from build123d import *

# Parameters (mm, degrees)
SLOT_DEPTH      = 26.980762114
SLOT_DEPTH_BACK = 26.980762114
SLOTSKE_W       = 3.5
SLOTSKE_H       = 1.8


with BuildPart() as part:
    # BodySke → Base-Revolve (revolve)
    with BuildSketch(Plane.XY, mode=Mode.PRIVATE) as base_revolve_sk:
        Polygon((0, 0), (0, 4), (1, 5), (24.172, 5), (25, 4.172), (25, 0), align=None)
    revolve(base_revolve_sk.sketch.rotate(Axis((-3.67611336, 0, 0), (1, 0, 0)), 90), axis=Axis((-3.67611336, 0, 0), (1, 0, 0)))

    # SlotSke → Slot (cut, two sides: drawn at the far end of the back side and taken through both)
    with BuildSketch(Plane.XY.offset(-SLOT_DEPTH_BACK)):
        with Locations((1.75, 0)):
            Rectangle(SLOTSKE_W, SLOTSKE_H)
    extrude(amount=SLOT_DEPTH + SLOT_DEPTH_BACK, mode=Mode.SUBTRACT)


solid = part.part
Could you check a few things on this model? Use its own coordinates, in mm. A direction names the side the tool comes from. Give positions to 0.01 mm unless a question says otherwise; leave off trailing zeros. Order: outer loops, then holes, each group sorted by start corner. A loop starts at its lowest first (then second) coordinate and runs counter-clockwise, first axis right, second up.
1. For faces 4 (the flat face through (25, 0, 0)), 5 (the flat face through (3.5, 0, 0)), which set-ups out of +Z, -Z, +X, -X, +Y, -Y let a thin tool reach every point of the face, with its end or its side?
2. Suppose I cut it at C-C (x = 20.25). List the corners of the cut face in (y, z) for me.
3. Will this pin go through, and if not, where does the flat tip stop? P1, Ø1.8, axis at x = 1, z = -0.5, coming from the -Y side.
4. Suppose I cut it at B-B (y = 0). List the corners of the cut face in (x, z) for me, plus the area to 3 significant figures.
5. Suppose I cut it at A-A (z = 0). List the corners of the cut face in (x, y) for me.
6. I need wall thicknesses on L1, parallel to X at y = 0, z = -1; L2, parallel to Y at x = 9.75, z = -3; L3, parallel to Y at x = 6.75, z = -0.25. Which ranges of each line are inside material? Lowest first, please.
7. We'd pull the mould along Y, two halves only. Please class faces 1 (the conical face through (0.2, 4.2, -0.1)), 2 (the flat face through (0, -2, 0)), 3 (the flat face through (2, 0.9, 0)): pulls with the +Y half, pulls with the -Y half, needs draft (parallel to the pull), parting line crosses it, or undercut.
Solved:
1. face 4: +Z, -Z, +X, +Y, -Y
1. face 5: +Z, -Z, -X
2. outline: circle Ø10 at (0, 0)
3. P1: stops at y = -5
4. outline: (3.5, -5) - (24.17, -5) - (25, -4.17) - (25, 4.17) - (24.17, 5) - (3.5, 5) - close
4. area: 214 mm2
5. outline: (0, -4) - (1, -5) - (24.17, -5) - (25, -4.17) - (25, 4.17) - (24.17, 5) - (1, 5) - (0, 4) - (0, 0.9) - (3.5, 0.9) - (3.5, -0.9) - (0, -0.9) - close
6. L1: x = 3.5 to 25
6. L2: y = -4 to 4
6. L3: y = -4.99 to 4.99
7. face 1: pulls with the +Y half
7. face 2: needs draft
7. face 3: undercut
